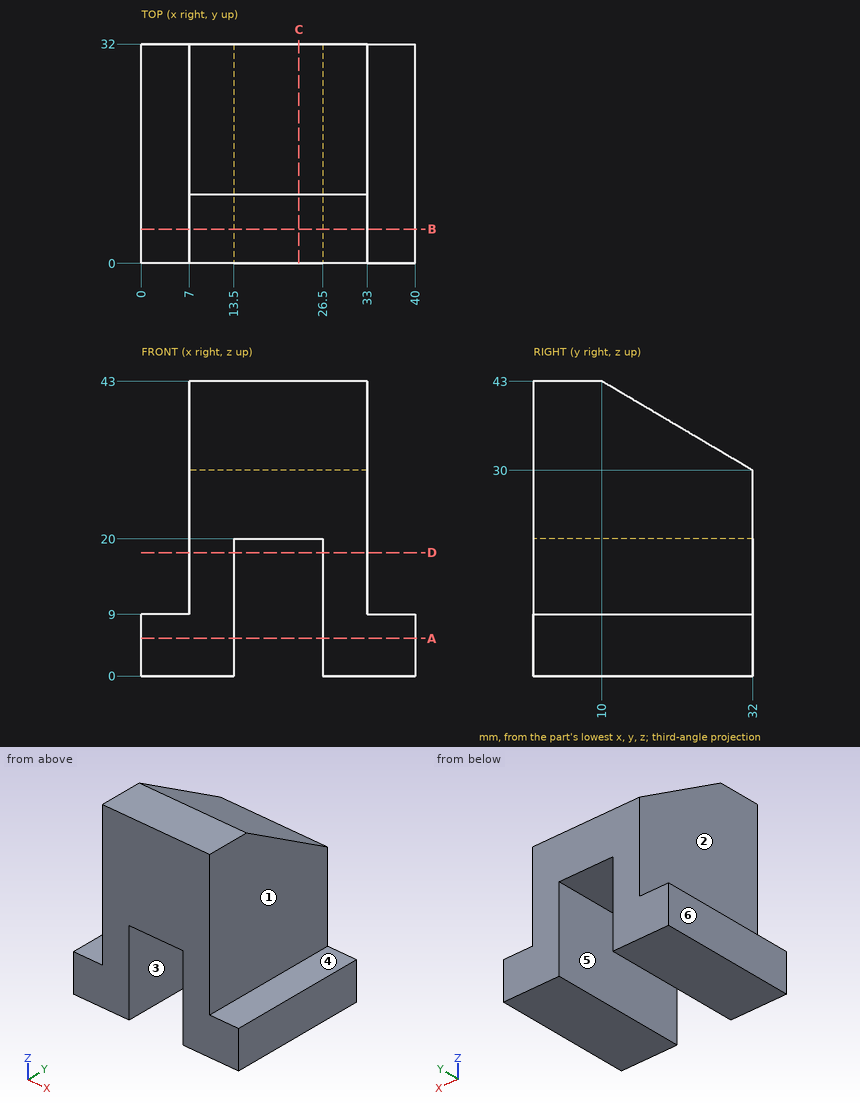
Check sheet for the drawn part. Datum: minimum x, y, z corner. Units: mm. A direction names the side the tool comes from. Round coordinates to 2 decimals unless told otherwise and drop trailing zeros. Loops run counter-clockwise (first coordinate to the right, second up) from the corner with the lowest first, then second, coordinate; pieces in that order, holes last. Notation, with made-up numbers: (49.5, 61.25) - (66.5, 61.25) arc R19 ccw to (66.5, 86.25) - close; hole circle Ø6 at (77, -28.75). An arc over 180 degrees is marked (long way). Answer as a JSON object with one key per item and string values. Group by question number.
Q1. Sectioned sample at A-A, the plane z = 5.5. Enter the section's corners in (x, y).
Q2. Mould release check, pull along X, two halves, no side actions. Record for the marked faces 4, 5 and 6: released by +X, released by -X, zero draft, split by the parting line, or undercut.
Q3. Scan lines: line 1 along X through (y, z) = (7.5, 13); line 2 along X through (y, z) = (25, 23.5); line 3 along Z through (x, y) = (2, 16.5). Record each from-to range of solid material in increasing order. Write a range as [from, to].
Q4. Sectioned sample at B-B, the plane y = 5. Enter the section's corners in (x, z).
Q5. Gauge pin test, flat ends, axial feed: P1, Ø1.5, axis at y = 9.5, z = 32.5, coming from the +X side; P2, Ø10, axis at x = 33.5, y = 25.5, coming from the +Z side; P3, Ø3.5, axis at x = 4.5, y = 16.5, coming from the +Z side; P4, Ø1, axis at x = 34.5, z = 30.5, coming from the -Y side. Record the tip position at first contact, or that the pin passes through.
Q6. Sectioned sample at C-C, the plane x = 23. Enter the section's corners in (y, z).
Q7. Set-up check for the marked faces 1, 2 and 3: record each of +Z, -Z, +X, -X, +Y, -Y from which the full face is reachable in a straight line by a thin tool's end or side.
Q8. Sectioned sample at D-D, the plane z = 18. Enter the section's corners in (x, y), plus the area to 3 significant figures.
Solution:
{
 "1": {"outline": "(0, 0) - (13.5, 0) - (13.5, 32) - (0, 32) - close; (26.5, 0) - (40, 0) - (40, 32) - (26.5, 32) - close"},
 "2": {"face 4": "zero draft", "face 5": "undercut", "face 6": "released by -X"},
 "3": {"line 1": "x = [7, 13.5], [26.5, 33]", "line 2": "x = [7, 33]", "line 3": "z = [0, 9]"},
 "4": {"outline": "(0, 0) - (13.5, 0) - (13.5, 20) - (26.5, 20) - (26.5, 0) - (40, 0) - (40, 9) - (33, 9) - (33, 43) - (7, 43) - (7, 9) - (0, 9) - close"},
 "5": {"P1": "stops at x = 33", "P2": "stops at z = 36.78", "P3": "stops at z = 9", "P4": "passes through"},
 "6": {"outline": "(0, 20) - (32, 20) - (32, 30) - (10, 43) - (0, 43) - close"},
 "7": {"face 1": "+Z, +X, +Y, -Y", "face 2": "+Z, -X, +Y, -Y", "face 3": "-Z, +Y, -Y"},
 "8": {"outline": "(7, 0) - (13.5, 0) - (13.5, 32) - (7, 32) - close; (26.5, 0) - (33, 0) - (33, 32) - (26.5, 32) - close", "area": "416 mm²"}
}
